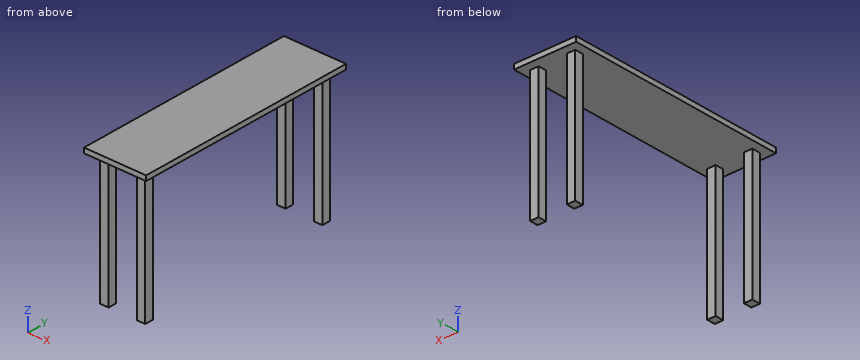
```python
from build123d import *

# Parameters (mm, degrees)
SKETCH1_W           = 558.8
SKETCH1_H           = 2006.6
BOSS_EXTRUDE1_DEPTH = 44.45
SKETCH5_W           = 76.2
SKETCH5_H           = 76.2
BOSS_EXTRUDE2_DEPTH = 1168.4


with BuildPart() as part:
    # Sketch1 → Boss-Extrude1 (new body)
    with BuildSketch(Plane.XY):
        Rectangle(SKETCH1_W, SKETCH1_H)
    extrude(amount=BOSS_EXTRUDE1_DEPTH)

    # Sketch5 → Boss-Extrude2 (add)
    with BuildSketch(Plane(origin=(0, 0, 0), x_dir=(-1, 0, 0), z_dir=(0, 0, -1))):
        with Locations((-165.1, 889)):
            Rectangle(SKETCH5_W, SKETCH5_H)
        with Locations((165.1, 889)):
            Rectangle(SKETCH5_W, SKETCH5_H)
        with Locations((-165.1, -889)):
            Rectangle(SKETCH5_W, SKETCH5_H)
        with Locations((165.1, -889)):
            Rectangle(SKETCH5_W, SKETCH5_H)
    extrude(amount=BOSS_EXTRUDE2_DEPTH)


solid = part.part
```
Geometry check sheet. Reference: the model listing, model coordinates, mm. Coordinates: 2 decimals unless noted, no trailing zeros. Write each loop counter-clockwise with the first axis right and the second up, starting at its lowest first coordinate (ties: lowest second). Pieces come first, ordered by that corner, then holes. Notation, with made-up numbers: M 85.5,-9 L 118.5,-9 A15 cw 118.5,19 Z; hole C -18,-20 d11. An arc over 180 degrees is marked long. Answer as a JSON object with one key per item and string values.
1. Section check A-A, the plane z = -525. Enter the section's corners in (x, y), plus the area to 3 significant figures.
Answers below:
{"outline": "M -203.2,-927.1 L -127,-927.1 L -127,-850.9 L -203.2,-850.9 Z; M -203.2,850.9 L -127,850.9 L -127,927.1 L -203.2,927.1 Z; M 127,-927.1 L 203.2,-927.1 L 203.2,-850.9 L 127,-850.9 Z; M 127,850.9 L 203.2,850.9 L 203.2,927.1 L 127,927.1 Z", "area": "23,200 mm²"}
2. Section check C-C, the plane y = 561. Enter the section's corners in (x, z).
Answers below:
{"outline": "M -279.4,0 L 279.4,0 L 279.4,44.45 L -279.4,44.45 Z"}
3. Go/stop test with flat-tipped pins: pin 1 Ø23 at (x, z) = (-161, -630.5) entering from -Y; pin 2 Ø23 at (y, z) = (900, -861.5) entering from -X. Record where each tip stops, or that it passes through.
Answers below:
{"pin 1": "stops at y = -927.1", "pin 2": "stops at x = -203.2"}
4. Scan lines: L1, parallel to Y at x = 138.5, z = -226.5; L2, parallel to X at y = 857, z = -217; L3, parallel to Z at x = -193, y = 723.5. Record each from-to range of solid material in increasing order.
Answers below:
{"L1": "y = -927.1 to -850.9, 850.9 to 927.1", "L2": "x = -203.2 to -127, 127 to 203.2", "L3": "z = 0 to 44.45"}
5. Section check B-B, the plane x = -80. Enter the section's corners in (y, z), plus the area to 3 significant figures.
Answers below:
{"outline": "M -1003.3,0 L 1003.3,0 L 1003.3,44.45 L -1003.3,44.45 Z", "area": "89,200 mm²"}
